from build123d import *

# Parameters (mm, degrees)
SKETCH1_R           = 3.99
BOSS_EXTRUDE1_DEPTH = 15
BOSS_EXTRUDE7_DEPTH = 15
SKETCH7_R           = 3.99
BOSS_EXTRUDE8_DEPTH = 25
SKETCH8_R           = 1.45
CUT_EXTRUDE1_DEPTH  = 8


with BuildPart() as part:
    # Sketch1 → Boss-Extrude1 (new body)
    with BuildSketch(Plane.XY):
        with Locations((-14.383915809, -0.854852817)):
            Circle(SKETCH1_R)
    extrude(amount=BOSS_EXTRUDE1_DEPTH)

    # Sketch6 → Boss-Extrude7 (add)
    with BuildSketch(Plane.XY.offset(15)):
        with BuildLine():
            Line((-17.383915809, 2.084534875), (-17.383915809, 8.084534875))
            Line((-17.383915809, 8.084534875), (-11.383915809, 8.084534875))
            Line((-11.383915809, 8.084534875), (-11.383915809, 2.084534875))
            ThreePointArc((-11.383915809, 2.084534875), (-14.383915809, -5.054852817), (-17.383915809, 2.084534875))
        make_face()
    extrude(amount=BOSS_EXTRUDE7_DEPTH)

    # Sketch7 → Boss-Extrude8 (add)
    with BuildSketch(Plane.XY.offset(30)):
        with Locations((-14.383915809, -0.854852817)):
            Circle(SKETCH7_R)
    extrude(amount=BOSS_EXTRUDE8_DEPTH)

    # Sketch8 → Cut-Extrude1 (cut)
    with BuildSketch(Plane(origin=(0, 8.084534875, 0), x_dir=(1, 0, 0), z_dir=(0, 1, 0))):
        with Locations((-14.343915809, -50)):
            Circle(SKETCH8_R)
    extrude(amount=-CUT_EXTRUDE1_DEPTH, mode=Mode.SUBTRACT)


solid = part.part
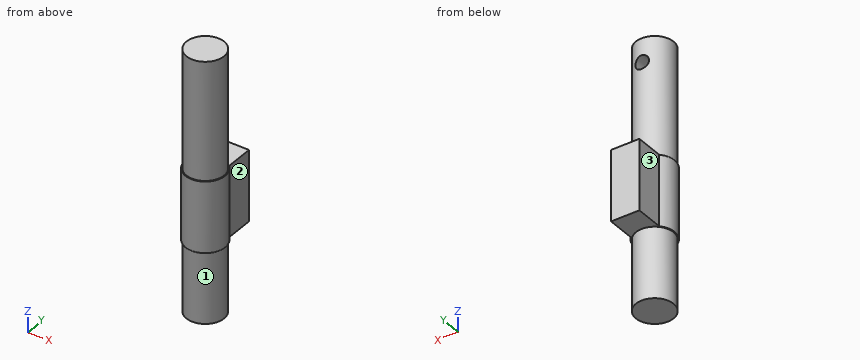
Model file for the job. Use its own axes, mm. Face numbers are marked on the shaded views. A direction names the side the tool comes from. Give positions to 0.01 mm unless a question says otherwise; leave off trailing zeros. Order: outer loops, then holes, each group sorted by start corner. A loop starts at its lowest first (then second) coordinate and runs counter-clockwise, first axis right, second up. Notation, with made-up numbers: (56.5, 24.25) - (86.5, 24.25) arc R21 ccw to (86.5, 45.25) - close; hole circle Ø6 at (8, 78.5). An arc over 180 degrees is marked (long way). Return JSON: item names as keys, results as strings.
1) Cut at A-A, the plane x = -13.5. Give the cut face in (y, z), plus the area to 3 significant figures.
Geometry says:
{"outline": "(-4.96, 15) - (-4.75, 15) - (-4.75, 0) - (3.04, 0) - (3.04, 15) - (8.08, 15) - (8.08, 30) - (3.04, 30) - (3.04, 48.82) - (0.08, 48.82) - (0.08, 51.18) - (3.04, 51.18) - (3.04, 55) - (-4.75, 55) - (-4.75, 30) - (-4.96, 30) - close", "area": "500 mm²"}
2) Cut at D-D, the plane z = 50. Give the cut face in (x, y), plus the area to 3 significant figures.
Geometry says:
{"outline": "(-15.79, 0.08) - (-15.79, 2.88) arc R3.99 ccw (long way) to (-12.89, 2.85) - (-12.89, 0.08) - close", "area": "41.4 mm²"}
3) Cut at B-B, the plane y = -2.75. Give the cut face in (x, z).
Geometry says:
{"outline": "(-18.13, 15) - (-17.9, 15) - (-17.9, 0) - (-10.87, 0) - (-10.87, 15) - (-10.64, 15) - (-10.64, 30) - (-10.87, 30) - (-10.87, 55) - (-17.9, 55) - (-17.9, 30) - (-18.13, 30) - close"}
4) Flat gauge pins, fed straight in: P1, Ø5, axis at y = -2, z = 44, coming from the -X side; P2, Ø5, axis at y = 6.5, z = 21, coming from the -X side; P3, Ø1, axis at y = 1, z = 40, coming from the +X side. Where does each tip first touch, or does it go through?
Geometry says:
{"P1": "x = -18.37", "P2": "x = -17.38", "P3": "x = -10.63"}
5) Cut at C-C, the plane z = 41. Give the cut face in (x, y), plus the area to 3 significant figures.
Geometry says:
{"outline": "circle Ø7.98 at (-14.38, -0.85)", "area": "50.0 mm²"}
6) 3-axis set-ups, long thin cutter, end or side, ignore diameter. For the marked faces 1, 2 and 3: which of +Z, -Z, +X, -X, +Y, -Y reach the whole face in a straight line?
Geometry says:
{"face 1": "-Z", "face 2": "+Z, -Z, +X, +Y", "face 3": "+Z, -Z, -X, +Y"}
7) Probe line 1 (X direction, y = 3.75, z = 18); line 2 (Z direction, x = -14.5, y = 5.5); line 3 (X direction, y = -1, z = 30.5). List the from-to ranges inside material, lowest first. Write a range as from..to.
Geometry says:
{"line 1": "-17.38..-11.38", "line 2": "15..30", "line 3": "-18.37..-10.4"}
